Can you work these out from the model? Positions are in its coordinate system, mm. A direction names the side the tool comes from. Give positions to 0.01 mm unless a question says otherwise; leave off trailing zeros. Order: outer loops, then holes, each group sorted by start corner. A loop starts at its lowest first (then second) coordinate and runs counter-clockwise, first axis right, second up. Notation, with made-up numbers: (32, 47.25) - (45, 47.25) arc R18 cw to (45, 77.25) - close; hole circle Ø9 at (-23.5, 6.25). An arc over 180 degrees is marked (long way). Return JSON: item names as keys, results as strings.
```python
from build123d import *

# Parameters (mm, degrees)
BOSS_EXTRUDE1_DEPTH     = 1754
FILLET2_R               = 3
CUT_EXTRUDE4_DEPTH      = 3
CUT_EXTRUDE4_DEPTH_BACK = 6
SKETCH8_W               = 30
SKETCH8_H               = 31


with BuildPart() as part:
    # Sketch3 → Boss-Extrude1 (new body)
    with BuildSketch(Plane(origin=(0, 0, 0), x_dir=(0, 0, -1), z_dir=(1, 0, 0))):
        Polygon((0, 0), (28, 0), (28, -28), (66, -28), (66, -81), (36, -81), (36, -78), (63, -78), (63, -31), (25, -31), (25, -3), (0, -3), align=None)
    extrude(amount=BOSS_EXTRUDE1_DEPTH)

    # Fillet2
    fillet2_edges = [part.edges().sort_by_distance(p)[0] for p in [
        (877, 0, -28),
        (877, -28, -28),
        (877, -28, -66),
        (877, -81, -66),
        (877, -78, -63),
        (877, -31, -63),
        (877, -31, -25),
        (877, -3, -25),
    ]]
    fillet(fillet2_edges, radius=FILLET2_R)

    # Sketch8 → Cut-Extrude4 (cut, two sides: drawn at the far end of the back side and taken through both)
    with BuildSketch(Plane(origin=(0, 0, -28), x_dir=(-1, 0, 0), z_dir=(0, 0, -1)).offset(-CUT_EXTRUDE4_DEPTH_BACK)):
        with Locations((-15, -15.5)):
            Rectangle(SKETCH8_W, SKETCH8_H)
        with Locations((-1739, -15.5)):
            Rectangle(SKETCH8_W, SKETCH8_H)
    extrude(amount=CUT_EXTRUDE4_DEPTH + CUT_EXTRUDE4_DEPTH_BACK, mode=Mode.SUBTRACT)


solid = part.part
```
1. For pin 1 Ø6.5 at (x, y) = (699, -18.5) entering from +Z; pin 2 Ø3.5 at (x, y) = (779, -80) entering from +Z; pin 3 Ø12 at (x, z) = (1213.5, -46.5) entering from +Y, each with a flat end and sliding along its axis, tell me the tip position at first contact or that it passes through.
Checks:
{"pin 1": "z = -25", "pin 2": "z = -36", "pin 3": "y = -28"}
2. Suppose I cut it at B-B (y = -53). List the corners of the cut face in (x, z) for me, plus the area to 3 significant figures.
Checks:
{"outline": "(0, -66) - (1754, -66) - (1754, -63) - (0, -63) - close", "area": "5,260 mm^2"}
3. On a 3-axis mill with a long thin cutter (end or side, diameter ignored), from which of +Z, -Z, +X, -X, +Y, -Y can I reach the whole of each face in a straight line? I mean faces 1 (the face through (1754, -48, -64)), 2 (the face through (865, -31, -44)), 3 (the face through (865, -28, -47)). Say none if no direction works.
Checks:
{"face 1": "+Z, -Z, +X, +Y, -Y", "face 2": "+Z, +X, -X", "face 3": "-Z, +X, -X, +Y"}
4. If I drill on L1, parallel to Y at x = 431, z = -14.5; L2, parallel to Z at x = 1245, y = -63.5; L3, parallel to Z at x = 414, y = -25, over which ranges is the centre line in solid material (lowest first)? Write a range as [from, to].
Checks:
{"L1": "[-3, 0]", "L2": "[-66, -63]", "L3": "[-28, -25]"}
5. Suppose I cut it at A-A (x = 696). List the corners of the cut face in (y, z) for me.
Checks:
{"outline": "(-81, -63) arc R3 ccw to (-78, -66) - (-31, -66) arc R3 ccw to (-28, -63) - (-28, -31) arc R3 cw to (-25, -28) - (-3, -28) arc R3 ccw to (0, -25) - (0, 0) - (-3, 0) - (-3, -22) arc R3 cw to (-6, -25) - (-28, -25) arc R3 ccw to (-31, -28) - (-31, -60) arc R3 cw to (-34, -63) - (-75, -63) arc R3 cw to (-78, -60) - (-78, -36) - (-81, -36) - close"}
6. Thinking about a two-plate mould opening in Y: for faces 4 (the face through (865, -55, -63)), 5 (the face through (865, -54, -66)), 6 (the face through (865, -81, -50)), which applies, +Y half, -Y half, draft (parallel to the pull), parting line (faces both ways), or undercut?
Checks:
{"face 4": "undercut", "face 5": "draft", "face 6": "-Y half"}
